```python
from build123d import *

# Parameters (mm, degrees)
F0_W        = 46.1472896859
F0_H        = 107.677012682
F1_DEPTH    = 5.334
F2_T1_DEPTH = 76.5470071681
F2_T3_DEPTH = 138.0767301641
F6_DEPTH    = 29.21
F8_DEPTH    = 30.226


# Not quite as in the source:
# - a fillet or chamfer that OpenCascade refuses, or shapes differently, is made with other operations: its cross-section is extruded or revolved along the edge and cut away or added
# - the program builds the solid bodies; features that only make, move or delete a surface that nothing else refers to are left out


with BuildPart() as f1:
    # F0 (on Front) → F1 (new body)
    with BuildSketch(Plane.XZ):
        with Locations((-8.118505124, 2.0296275616)):
            Rectangle(F0_W, F0_H)
    extrude(amount=F1_DEPTH)

    # F2: fillet of radius 6.1321024484 on 4 edges, made by hand

    # F2_s2 → F2_t1 (cut)
    with BuildSketch(Plane.YZ.offset(-46.392008708)):
        with BuildLine():
            ThreePointArc((0, 55.8681339025), (-3.8114922418, 53.8322375411), (-5.334, 49.7881904061))
            Line((-5.334, 49.7881904061), (-5.334, 55.8681339025))
            Line((-5.334, 55.8681339025), (0, 55.8681339025))
        make_face()
        with BuildLine():
            ThreePointArc((0, -51.8088787794), (-3.8114922418, -49.772982418), (-5.334, -45.728935283))
            Line((-5.334, -45.728935283), (-5.334, -51.8088787794))
            Line((-5.334, -51.8088787794), (0, -51.8088787794))
        make_face()
    extrude(amount=F2_T1_DEPTH, mode=Mode.SUBTRACT)

    # F2_s4 → F2_t3 (cut)
    with BuildSketch(Plane.XY.offset(-67.0087375205)):
        with BuildLine():
            ThreePointArc((-31.192149967, 0), (-29.1562536055, -3.8114922418), (-25.1122064705, -5.334))
            Line((-25.1122064705, -5.334), (-31.192149967, -5.334))
            Line((-31.192149967, -5.334), (-31.192149967, 0))
        make_face()
        with BuildLine():
            ThreePointArc((14.9551397189, 0), (12.9192433575, -3.8114922418), (8.8751962225, -5.334))
            Line((8.8751962225, -5.334), (14.9551397189, -5.334))
            Line((14.9551397189, -5.334), (14.9551397189, 0))
        make_face()
    extrude(amount=F2_T3_DEPTH, mode=Mode.SUBTRACT)

    # F5 (on Front) → F6 (join)
    with BuildSketch(Plane.XZ):
        Polygon((-25.2416264266, 49.8663634062), (-28.8135651499, 49.8663634062), (-29.4354222715, 44.9747443199), (-25.2416264266, 44.9747443199), align=None)
    extrude(amount=-F6_DEPTH)

    # F7 (on Front) → F8 (join)
    with BuildSketch(Plane.XZ):
        Polygon((11.3538028672, -49.219802022), (11.3571733236, -43.9655184746), (7.279606536, -43.9655184746), (7.279606536, -49.219802022), align=None)
    extrude(amount=-F8_DEPTH)


solid = f1.part
```
Read the model definition and answer for the solid it produces. Units are mm, in the model's axes. A direction names the side the tool comes from. Coordinates: 2 decimals unless noted, no trailing zeros. Write each loop counter-clockwise with the first axis right and the second up, starting at its lowest first coordinate (ties: lowest second). Pieces come first, ordered by that corner, then holes. Notation, with made-up numbers: (-21.5, 65.5) - (-9.5, 65.5) arc R15 ccw to (-9.5, 90.5) - close; hole circle Ø4 at (13, 63.25). An arc over 180 degrees is marked (long way). Answer as a JSON object with one key per item and string values. Group by question number.
1. A cutting plane is placed at A-A (y = 3). Determine the outline of the cut face in (x, z).
2. A cutting plane is placed at C-C (x = -19). Determine the outline of the cut face in (y, z), plus the area to 3 significant figures.
3. A cutting plane is placed at D-D (z = 47.5). Determine the outline of the cut face in (x, y), plus the area to 3 significant figures.
4. Which of the six approach directions +Z, -Z, +X, -X, +Y, -Y give full straight-line access (tool end or side, diameter ignored) to faces 1 (the flat face through (9, 15, -43.966)), 2 (the flat face through (9, 15, -49.22)), 3 (the flat face through (-25.242, 14, 47)), 4 (the flat face through (-29.12, 14.4, 47.45))?
5. Each of these flat-tipped pins is pushed along its axis until it touches: P1, Ø4, axis at y = 18, z = 46.5, coming from the +X side; P2, Ø8, axis at y = 1.5, z = 4.5, coming from the -X side; P3, Ø2, axis at x = -25.5, y = 11, coming from the -Z side. Where does it stop, or does it pass through?
6. A cutting plane is placed at B-B (z = 18). Determine the outline of the cut face in (x, y), plus the area to 3 significant figures.
7. Consider L1, parallel to Z at x = -25.5, y = 16; L2, parallel to Y at x = 8.5, z = 28.5; L3, parallel to Y at x = -27, z = 47. Determine where each line is inside the solid, lowest interval first. Write a range as [from, to].
Worked out:
{
 "1": {"outline": "(-29.44, 44.97) - (-25.24, 44.97) - (-25.24, 49.87) - (-28.81, 49.87) - close; (7.28, -49.22) - (11.35, -49.22) - (11.36, -43.97) - (7.28, -43.97) - close"},
 "2": {"outline": "(-5.33, -45.73) arc R6.13 ccw to (0, -51.81) - (0, 55.87) arc R6.13 ccw to (-5.33, 49.79) - close", "area": "559 mm²"},
 "3": {"outline": "(-31.19, 0) arc R6.13 ccw to (-25.11, -5.33) - (8.88, -5.33) arc R6.13 ccw to (14.96, 0) - (-25.24, 0) - (-25.24, 29.21) - (-29.11, 29.21) - (-29.11, 0) - close", "area": "344 mm²"},
 "4": {"face 1": "+Z, +X, -X, +Y", "face 2": "-Z, +X, -X, +Y", "face 3": "+Z, -Z, +X, +Y", "face 4": "+Z, -X, +Y"},
 "5": {"P1": "stops at x = -25.24", "P2": "stops at x = -31.19", "P3": "stops at z = 44.97"},
 "6": {"outline": "(-31.19, 0) arc R6.13 ccw to (-25.11, -5.33) - (8.88, -5.33) arc R6.13 ccw to (14.96, 0) - close", "area": "231 mm²"},
 "7": {"L1": "z = [44.97, 49.87]", "L2": "y = [-5.33, 0]", "L3": "y = [-5.04, 29.21]"}
}
